Geometry: see drawing. Coordinates: mm, zero at the bounding-box minimum. Coordinates: 2 decimals unless noted, no trailing zeros. Write each loop counter-clockwise with the first axis right and the second up, starting at its lowest first coordinate (ties: lowest second). Pieces come first, ordered by that corner, then holes. Notation, with made-up numbers: M 60,-21 L 104,-21 A4 ccw 104,-16 Z; hole C 24,76 d9. An arc over 180 degrees is marked long. Write item = value, one per line. Start each with the question number.
1. Pin query (flat end, axial travel): pin 1 Ø2.5 at (x, z) = (55, 20) entering from +Y. Return the tip coordinate at first contact, or that it passes through.
2. Section query B-B (z = 20). Output: boundary loops of the cut face in (x, y), then the cut area to 3 significant figures.
3. Line query: line 1 along Z through (x, y) = (55, 1.25); line 2 along X through (y, z) = (2.85, 19.5). Output: solid intervals per line, ascending.
4. Section query A-A (x = 80). Output: boundary loops of the cut face in (y, z), then the cut area to 3 significant figures.
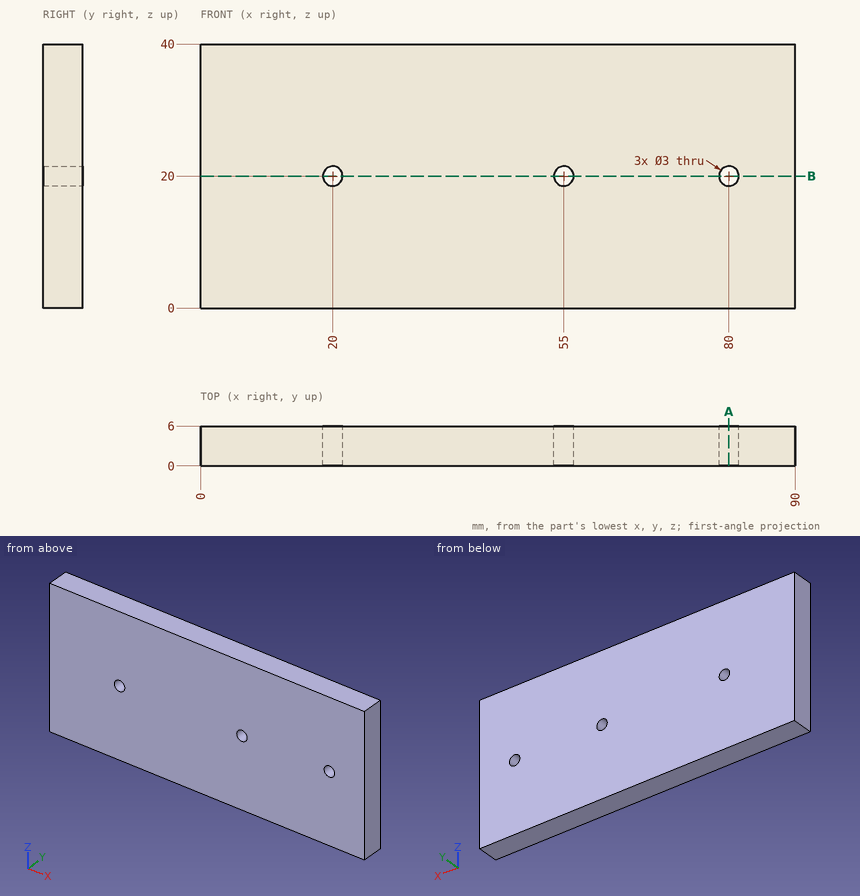
Results are:
q1.pin_1 = through
q2.outline = M 0,0 L 18.5,0 L 18.5,6 L 0,6 Z; M 21.5,0 L 53.5,0 L 53.5,6 L 21.5,6 Z; M 56.5,0 L 78.5,0 L 78.5,6 L 56.5,6 Z; M 81.5,0 L 90,0 L 90,6 L 81.5,6 Z
q2.area = 486 mm^2
q3.line_1 = 0 to 18.5, 21.5 to 40
q3.line_2 = 0 to 18.59, 21.41 to 53.59, 56.41 to 78.59, 81.41 to 90
q4.outline = M 0,0 L 6,0 L 6,18.5 L 0,18.5 Z; M 0,21.5 L 6,21.5 L 6,40 L 0,40 Z
q4.area = 222 mm^2
